Autodesk Inventor part; units mm, degrees
ref_plane "YZ Plane" through (0, 0, 0) normal (1, 0, 0) x (0, 1, 0)
ref_plane "XZ Plane" through (0, 0, 0) normal (0, 1, 0) x (-1, 0, 0)
ref_plane "XY Plane" through (0, 0, 0) normal (0, 0, 1) x (1, 0, 0)
sketch "Sketch1" plane through (0, 0, 0) normal (1, 0, 0) x (0, 1, 0)
  line L0 (-116.2182, 0) -> (19.3697, 0)
  line L1 (-46.9485, -33.2) -> (-46.9485, -41.2)
  line L2 (-11.4485, -41.2) -> (-46.9485, -41.2)
  line L3 (-48.3, -33.2) -> (-60.6, -33.2)
  line L4 (-11.4485, -42.2) -> (-48.9485, -42.2)
  line L5 (-48.9485, -42.2) -> (-48.9485, -35.2)
  line L6 (-48.9485, -35.2) -> (-96.8485, -35.2)
  line L7 (-96.8485, -35.2) -> (-96.8485, -33.2)
  line L8 (-46.9485, -33.2) -> (-48.3, -33.2)
  line L9 (-63.9485, -33.2) -> (-63.9485, -30.2)
  line L10 (-63.9485, -30.2) -> (-65.9485, -30.2)
  line L11 (-65.9485, -30.2) -> (-65.9485, -33.2)
  line L12 (-96.8485, -33.2) -> (-65.9485, -33.2)
  line L13 (-63.9485, -33.2) -> (-60.6, -33.2)
  line L14 (-11.4485, -41.2) -> (-11.4485, -42.2)
  point P0 (0, 0)
  point P1 (-46.9485, -41.7)
  point P2 (-96.8485, -34.2)
  point P3 (-48.9485, -38.7)
  point P4 (-11.4485, -41.7)
  dimension "d43" = 41.2
  dimension "d53" = 33.2
  dimension "d58" = 1
  dimension "d61" = 2
  dimension "d65" = 2
  dimension "d66" = 17
  dimension "d68" = 49.9
  dimension "d69" = 35.5
  dimension "d72" = 2
  dimension "d74" = 42.2
  dimension "d78" = 35.5
  dimension "d79" = 3
revolve "Revolution1" add sketch "Sketch1" angle 360 about axis through (0, -10, 0) along (0, 1, 0)
sketch "Sketch2" plane through (0, 0, 0) normal (1, 0, 0) x (0, 1, 0)
  line L0 (-96.8485, -35.2) -> (-96.8485, 35.2)
  line L1 (-114.1482, 0) -> (19.0247, 0)
  point P0 (0, 0)
  point P1 (-55.4485, 0)
  dimension "d64" = 41.4
hole "Hole1" at (0, -55.4485, 0) direction (1, 0, 0) diameter 1.9 depth 40
hole "Hole2" at (0, -55.4485, 0) direction (-1, 0, 0) diameter 1.9 depth 40
fillet "Fillet1" [suppressed]
fillet "Fillet3" radius 3 1 edges at (0, -65.9485, 33.2)
equation "\"gap\" = 0.1"
properties part number "BottomTubeDown"
The model under review builds one solid part; all positions refer to its coordinate system, in mm. A direction names the side the tool comes from. Give positions to 0.01 mm unless a question says otherwise; leave off trailing zeros. Write each loop counter-clockwise with the first axis right and the second up, starting at its lowest first coordinate (ties: lowest second). Pieces come first, ordered by that corner, then holes. Notation, with made-up numbers: (2.5, 53.25) -> (57.5, 53.25) arc R10 ccw to (57.5, 72.25) -> close; hole circle Ø3 at (42.5, 1). An arc over 180 degrees is marked (long way). Answer in a Markdown table with one row per item.
1) Clearance check with flat-ended pins moving along their axes: P1, Ø12, axis at y = -46, z = -28, coming from the -X side; P2, Ø1.5, axis at x = -27, y = -33, coming from the +Z side; P3, Ø4, axis at y = -24, z = -4.5, coming from the +X side; P4, Ø1.7, axis at y = -55.45, z = 0, coming from the +X side. State where each tip first meets the part, or that it passes through.
Worked answers:
| item | result |
|---|---|
| P1 | x = -36.01 |
| P2 | z = 33.04 |
| P3 | x = 42.13 |
| P4 | through |
2) Tool access review of faces 4 (the flat face through (40.4, -11.448, -9.2)), 5 (the cylindrical face through (32.41, -82.7, 7.2)), 6 (the cylindrical face through (-32.41, -55.57, 7.2)): name each direction out of +Z, -Z, +X, -X, +Y, -Y from which nothing blocks a thin tool from reaching the whole face with its end or side.
Worked answers:
| item | result |
|---|---|
| face 4 | +Z, -Z, +X, -X, +Y |
| face 5 | -Y |
| face 6 | +Y |
3) For L1, parallel to Y at x = -33.85, z = 0; L2, parallel to X at y = -59, z = 0, list the stretches that pass through material, from the lowest coordinate up. Write a range as [from, to].
Worked answers:
| item | result |
|---|---|
| L1 | [-96.85, -56.4], [-54.5, -46.95] |
| L2 | [-35.2, -33.2], [33.2, 35.2] |
4) Add section C-C on y = -30. State the section outline as (x, z) points.
Worked answers:
| item | result |
|---|---|
| outline | circle Ø84.4 at (0, 0); hole circle Ø82.4 at (0, 0) |
5) Add section B-B on y = -82. State the section outline as (x, z) points, plus the area to 3 significant figures.
Worked answers:
| item | result |
|---|---|
| outline | circle Ø70.4 at (0, 0); hole circle Ø66.4 at (0, 0) |
| area | 430 mm² |
6) Mouldability with a two-part tool opening along Z and no side actions: class faces 1 (the cylindrical face through (-29.48, -64.96, 6.55)), 2 (the flat face through (26, -96.848, 21)), 3 (the cylindrical face through (10.573, -73.234, -33.575)) as +Z half, -Z half, draft (parallel to the pull), parting line (faces both ways), or undercut.
Worked answers:
| item | result |
|---|---|
| face 1 | undercut |
| face 2 | draft |
| face 3 | parting line |
